from build123d import *

# Parameters (mm, degrees)
F1_DEPTH = 28.575
F2_DEPTH = 14.2875
F3_DEPTH = 14.2875
F4_R     = 5.08
F5_DEPTH = 9.525
F6_SIZE  = 7.62


with BuildPart() as f1:
    # F0 (on Front) → F1 (new body, symmetric)
    with BuildSketch(Plane.XZ):
        with BuildLine():
            Line((-32.86058, -11.644275), (-32.86058, -25.442014))
            Line((-32.86058, -25.442014), (27.46442, -25.442014))
            Line((27.46442, -25.442014), (27.46442, -19.346014))
            ThreePointArc((27.46442, -19.346014), (43.33942, -3.471014), (59.21442, -19.346014))
            Line((59.21442, -19.346014), (59.21442, -25.442014))
            Line((59.21442, -25.442014), (78.26442, -25.442014))
            Line((78.26442, -25.442014), (78.26442, -18.228882))
            Line((78.26442, -18.228882), (78.26442, -12.742014))
            Line((78.26442, -12.742014), (65.56442, -12.742014))
            Line((65.56442, -12.742014), (65.56442, 9.482986))
            Line((65.56442, 9.482986), (37.893278, 9.482986))
            Line((37.893278, 9.482986), (21.11442, 9.482986))
            Line((21.11442, 9.482986), (21.11442, -12.742014))
            Line((21.11442, -12.742014), (-29.68558, -12.742014))
            Line((-29.68558, -12.742014), (-29.68558, 9.482986))
            Line((-29.68558, 9.482986), (-42.38558, 9.482986))
            Line((-42.38558, 9.482986), (-42.38558, 14.788094))
            Line((-42.38558, 14.788094), (-42.38558, 20.093201))
            Line((-42.38558, 20.093201), (-64.61058, 20.093201))
            Line((-64.61058, 20.093201), (-64.61058, 13.743201))
            Line((-64.61058, 13.743201), (-60.467657, 10.428858))
            Line((-60.467657, 10.428858), (-60.467657, -14.971142))
            Line((-60.467657, -14.971142), (-55.692457, -14.971142))
            Line((-55.692457, -14.971142), (-53.014755, -6.6675))
            Line((-53.014755, -6.6675), (-37.139755, -6.6675))
            Line((-37.139755, -6.6675), (-32.86058, -11.644275))
        make_face()
    extrude(amount=F1_DEPTH, both=True)

    # F0 (on Front) → F2 (join, symmetric)
    with BuildSketch(Plane.XZ):
        Polygon((21.11442, -12.742014), (21.11442, 9.482986), (-21.76078, 9.690133), (-29.68558, 9.482986), (-29.68558, -12.742014), align=None)
    extrude(amount=F2_DEPTH, both=True)

    # F0 (on Front) → F3 (join, symmetric)
    with BuildSketch(Plane.XZ):
        Polygon((-21.76078, 14.788094), (-42.38558, 14.788094), (-42.38558, 9.482986), (-29.68558, 9.482986), (-21.76078, 9.690133), align=None)
    extrude(amount=F3_DEPTH, both=True)

    # F4
    f4_edges = [f1.edges().sort_by_distance(p)[0] for p in [
        (65.56442, 0, 9.482986),
    ]]
    fillet(f4_edges, radius=F4_R)

    # F0 (on Front) → F5 (join, symmetric)
    with BuildSketch(Plane.XZ):
        with BuildLine():
            Line((21.11442, 9.482986), (37.893278, 9.482986))
            Line((37.893278, 9.482986), (22.453869, 21.300806))
            ThreePointArc((22.453869, 21.300806), (21.02995, 22.122689), (19.442752, 22.551457))
            Line((19.442752, 22.551457), (3.988611, 24.635159))
            ThreePointArc((3.988611, 24.635159), (0.087031, 24.757666), (-3.75761, 24.082341))
            Line((-3.75761, 24.082341), (-17.814589, 20.093201))
            Line((-17.814589, 20.093201), (-21.76078, 14.788094))
            Line((-21.76078, 14.788094), (-21.76078, 9.690133))
            Line((-21.76078, 9.690133), (21.11442, 9.482986))
        make_face()
    extrude(amount=F5_DEPTH, both=True)

    # F6
    f6_edges = [f1.edges().sort_by_distance(p)[0] for p in [
        (78.26442, -28.575, -19.092014),
        (78.26442, 28.575, -19.092014),
    ]]
    chamfer(f6_edges, length=F6_SIZE)


solid = f1.part
Source: CAD feature listing. Evaluate the final solid. Frame: model axes, mm. A direction names the side the tool comes from. Give positions to 0.01 mm unless a question says otherwise; leave off trailing zeros. Write each loop counter-clockwise with the first axis right and the second up, starting at its lowest first coordinate (ties: lowest second). Pieces come first, ordered by that corner, then holes. Notation, with made-up numbers: (-20.5, 16) - (37.5, 16) arc R16 cw to (37.5, 29) - close; hole circle Ø8 at (9, -1.75). An arc over 180 degrees is marked (long way). Write item = value, one per line. Start each with the question number.
Q1. Pin query (flat end, axial travel): pin 1 Ø7 at (y, z) = (-24.5, -6) entering from -X; pin 2 Ø10 at (x, y) = (-37, -19) entering from +Z; pin 3 Ø7 at (x, y) = (-3, 19.5) entering from +Z. Return the tip coordinate at first contact, or that it passes through.
Q2. Cut plane B-B, the plane z = -17. Return loops of the section in (x, y) (3 decimals).
Q3. Material intervals for probe 1 along X at (y, z) = (-16.5, -7.5); probe 2 along X at (y, z) = (-23.5, -8.5); probe 3 along X at (y, z) = (-4, -11), sorted ascending.
Q4. Cut plane C-C, the plane x = -9. Return loops of the section in (y, z) (1 decimal).
Q5. Reachability of faces 4 (the flat face through (8, -9.525, 16)), 5 (the flat face through (72, 0, -12.742)), 6 (the flat face through (-29.686, -22, -2)), 7 (the flat face through (-60.468, 0, -2)) from +Z, -Z, +X, -X, +Y, -Y: full face, straight path, thin tool, end or side. Return the list, or none.
Q6. Cut plane D-D, the plane x = 30. Return loops of the section in (y, z) (3 decimals), then the cut area to 3 significant figures.
Q7. Draft query along X for faces 1 (the flat face through (11.82, -0.13, 23.58)), 2 (the flat face through (-36, -22, 9.483)), 3 (the flat face through (-45, 0, -6.668)). Return one class per face: +X half, -X half, draft (parallel to the pull), parting line (faces both ways), or undercut.
Computed values:
q1.pin_1 = -60.47
q1.pin_2 = 14.79
q1.pin_3 = -12.74
q2.outline = (-32.861, -28.575) - (27.639, -28.575) - (27.639, 28.575) - (-32.861, 28.575) - close; (59.04, -28.575) - (70.644, -28.575) - (78.264, -20.955) - (78.264, 20.955) - (70.644, 28.575) - (59.04, 28.575) - close
q3.probe_1 = -60.47 to -53.28, -36.42 to -29.69, 21.11 to 32.77, 53.91 to 65.56
q3.probe_2 = -60.47 to -53.61, -35.56 to -29.69, 21.11 to 31.75, 54.93 to 65.56
q3.probe_3 = -60.47 to -54.41, -33.41 to 29.84, 56.84 to 65.56
q4.outline = (-28.6, -25.4) - (28.6, -25.4) - (28.6, -12.7) - (14.3, -12.7) - (14.3, 9.6) - (9.5, 9.6) - (9.5, 22.6) - (-9.5, 22.6) - (-9.5, 9.6) - (-14.3, 9.6) - (-14.3, -12.7) - (-28.6, -12.7) - close
q5.face_4 = +Z, +X, -Y
q5.face_5 = +Z, +X, +Y, -Y
q5.face_6 = +Z, -Y
q5.face_7 = -Z, -X, +Y, -Y
q6.outline = (-28.575, -10.739) - (28.575, -10.739) - (28.575, 9.483) - (9.525, 9.483) - (9.525, 15.525) - (-9.525, 15.525) - (-9.525, 9.483) - (-28.575, 9.483) - close
q6.area = 1,270 mm²
q7.face_1 = +X half
q7.face_2 = draft
q7.face_3 = undercut
